from build123d import *

# Parameters (mm, degrees)
PAD_DEPTH       = 25
SKETCH001_R     = 4.3
POCKET_DEPTH    = 20.001
POCKET001_DEPTH = 15.001
FILLET_R        = 4
FILLET001_R     = 18


with BuildPart() as part:
    # Sketch → Pad (new body)
    with BuildSketch(Plane.XZ):
        with BuildLine():
            Line((40.4, -5.4), (65.4, -5.4))
            Line((65.4, -5.4), (65.4, -15.4))
            Line((26.4, -25.4), (65.4, -15.4))
            Line((-26.4, -25.4), (26.4, -25.4))
            Line((-65.4, -15.4), (-26.4, -25.4))
            Line((-65.4, -15.4), (-65.4, -5.4))
            Line((-65.4, -5.4), (-40.4, -5.4))
            Line((-40.4, -6.4), (-40.4, -5.4))
            ThreePointArc((-26.4, -20.4), (-30.500505, -10.500505), (-40.4, -6.4))
            Line((-26.4, -20.4), (26.4, -20.4))
            ThreePointArc((40.4, -6.4), (30.500505, -10.500505), (26.4, -20.4))
            Line((40.4, -6.4), (40.4, -5.4))
        make_face()
    extrude(amount=PAD_DEPTH)

    # Sketch001 (on Face8 of Pad) → Pocket (cut, through all)
    with BuildSketch(Plane(origin=(0, 0, -5.4), x_dir=(-1, 0, 0), z_dir=(0, 0, 1))):
        with Locations((-52.9, 12.5)):
            Circle(SKETCH001_R)
        with Locations((52.9, 12.5)):
            Circle(SKETCH001_R)
    extrude(amount=-POCKET_DEPTH, mode=Mode.SUBTRACT)

    # Sketch002 (on Face13 of Pocket) → Pocket001 (cut, through all)
    with BuildSketch(Plane(origin=(0, 0, -10.4), x_dir=(-1, 0, 0), z_dir=(0, 0, 1))):
        Polygon((-46.3, 8.689488), (-46.3, 16.310512), (-52.9, 20.121024), (-59.5, 16.310512), (-59.5, 8.689488), (-52.9, 4.878976), align=None)
        Polygon((59.5, 8.689488), (59.5, 16.310512), (52.9, 20.121024), (46.3, 16.310512), (46.3, 8.689488), (52.9, 4.878976), align=None)
    extrude(amount=-POCKET001_DEPTH, mode=Mode.SUBTRACT)

    # Fillet
    fillet_edges = [part.edges().sort_by_distance(p)[0] for p in [
        (-65.4, -25, -10.4),
        (-65.4, 0, -10.4),
        (65.4, -25, -10.4),
        (65.4, 0, -10.4),
    ]]
    fillet(fillet_edges, radius=FILLET_R)

    # Fillet001
    fillet001_edges = [part.edges().sort_by_distance(p)[0] for p in [
        (-26.4, -12.5, -25.4),
        (26.4, -12.5, -25.4),
    ]]
    fillet(fillet001_edges, radius=FILLET001_R)


solid = part.part
Verification items for the finished model (mm, model axes). A direction names the side the tool comes from. Coordinates: 2 decimals unless noted, no trailing zeros. Order: outer loops, then holes, each group sorted by start corner. A loop starts at its lowest first (then second) coordinate and runs counter-clockwise, first axis right, second up.
Item 1: Section check A-A, the plane y = -12.5. Give the number of separate pieces and of enclosed holes in the cut face, then the cut area to 3 significant figures.
Filled in:
separate pieces: 3
enclosed holes: 0
area: 1,020 mm2
Item 2: Section check D-D, the plane x = 55.5. Enter the section's corners in (y, z), then the cut area to 3 significant figures.
Filled in:
outline: (-25, -17.94) - (-18.62, -17.94) - (-18.62, -10.4) - (-15.92, -10.4) - (-15.92, -5.4) - (-25, -5.4) - close; (-9.08, -10.4) - (-6.38, -10.4) - (-6.38, -17.94) - (0, -17.94) - (0, -5.4) - (-9.08, -5.4) - close
area: 187 mm2
Item 3: Section check B-B, the plane z = -9.25. Enter the section's corners in (x, y), then the cut area to 3 significant figures.
Filled in:
outline: (-65.4, -21) arc R4 ccw to (-61.4, -25) - (-31.93, -25) - (-31.93, 0) - (-61.4, 0) arc R4 ccw to (-65.4, -4) - close; (31.93, -25) - (61.4, -25) arc R4 ccw to (65.4, -21) - (65.4, -4) arc R4 ccw to (61.4, 0) - (31.93, 0) - close; hole circle Ø8.6 at (-52.9, -12.5); hole circle Ø8.6 at (52.9, -12.5)
area: 1,540 mm2
Item 4: Material ranges on L1, parallel to Y at x = 52.9, z = -8.2; L2, parallel to X at y = -12.5, z = -8.65; L3, parallel to X at y = -6.5, z = -11, recorded low to high.
Filled in:
L1: y = -25 to -16.8, -8.2 to 0
L2: x = -65.4 to -57.2, -48.6 to -32.79, 32.79 to 48.6, 57.2 to 65.4
L3: x = -65.4 to -55.71, -50.09 to -30.03, 30.03 to 50.09, 55.71 to 65.4
Item 5: Section check C-C, the plane x = -56. Enter the section's corners in (y, z).
Filled in:
outline: (-25, -17.81) - (-18.33, -17.81) - (-18.33, -10.4) - (-15.48, -10.4) - (-15.48, -5.4) - (-25, -5.4) - close; (-9.52, -10.4) - (-6.67, -10.4) - (-6.67, -17.81) - (0, -17.81) - (0, -5.4) - (-9.52, -5.4) - close
Item 6: Depth check by flat-ended pin: pin 1 (1 mm diameter, centred on x = -10.5, y = -15, fed in from +Z); pin 2 (11 mm diameter, centred on x = 52.9, y = -12.5, fed in from -Z); pin 3 (6 mm diameter, centred on y = -11, z = -15.5, fed in from +X); pin 4 (1 mm diameter, centred on x = 35.5, y = -17, fed in from -Z). Enter the tip coordinate at first touch or a pass-through.
Filled in:
pin 1: stops at z = -20.4
pin 2: stops at z = -10.4
pin 3: stops at x = 65.4
pin 4: stops at z = -23.19
Item 7: Access from +Z, -Z, +X, -X, +Y, -Y to the whole of each face (thin tool, end or side, straight path). Record for faces 1 (the face through (-26.351, -12.675, -25.262)), 2 (the face through (-50, -9, -10.4)), 3 (the face through (30.6, -12.3, -10.4)).
Filled in:
face 1: -Z, -X, +Y, -Y
face 2: -Z
face 3: +Z, +Y, -Y
Item 8: Release check for a two-part mould opening along Y. For faces 4 (the face through (57.196, -12.689, -7.865)), 5 (the face through (1, -25, -22)), 6 (the face through (0, -12, -25.4)) record: +Y half, -Y half, draft (parallel to the pull), parting line (faces both ways), or undercut.
Filled in:
face 4: undercut
face 5: -Y half
face 6: draft
